```python
from build123d import *

# Parameters (mm, degrees)
SKETCH1_W           = 76.2
SKETCH1_H           = 25.4
BOSS_EXTRUDE1_DEPTH = 6.35
SKETCH2_W           = 76.2
SKETCH2_H           = 25.4
BOSS_EXTRUDE2_DEPTH = 6.35
FILLET1_R           = 3.175
FILLET2_R           = 2.3876
SKETCH3_R           = 3.3782
CUT_EXTRUDE1_DEPTH  = 7.35
SKETCH4_R           = 3.3782
CUT_EXTRUDE2_DEPTH  = 7.35


with BuildPart() as part:
    # Sketch1 → Boss-Extrude1 (new body)
    with BuildSketch(Plane(origin=(0, 0, 0), x_dir=(1, 0, 0), z_dir=(0, 1, 0))):
        with Locations((38.1, 12.7)):
            Rectangle(SKETCH1_W, SKETCH1_H)
    extrude(amount=BOSS_EXTRUDE1_DEPTH)

    # Sketch2 → Boss-Extrude2 (add)
    with BuildSketch(Plane(origin=(0, 0, -25.4), x_dir=(-1, 0, 0), z_dir=(0, 0, -1))):
        with Locations((-38.1, 12.7)):
            Rectangle(SKETCH2_W, SKETCH2_H)
    extrude(amount=-BOSS_EXTRUDE2_DEPTH)

    # Fillet1
    fillet1_edges = [part.edges().sort_by_distance(p)[0] for p in [
        (38.1, 6.35, -19.05),
    ]]
    fillet(fillet1_edges, radius=FILLET1_R)

    # Fillet2
    fillet2_edges = [part.edges().sort_by_distance(p)[0] for p in [
        (38.1, 25.4, -19.05),
        (38.1, 6.35, 0),
    ]]
    fillet(fillet2_edges, radius=FILLET2_R)

    # Sketch3 → Cut-Extrude1 (cut, through all)
    with BuildSketch(Plane(origin=(0, 6.35, 0), x_dir=(1, 0, 0), z_dir=(0, 1, 0))):
        with Locations((13.21308, 9.1313)):
            Circle(SKETCH3_R)
        with Locations((29.80436, 9.1313)):
            Circle(SKETCH3_R)
        with Locations((46.39564, 9.1313)):
            Circle(SKETCH3_R)
        with Locations((62.98692, 9.1313)):
            Circle(SKETCH3_R)
    extrude(amount=-CUT_EXTRUDE1_DEPTH, mode=Mode.SUBTRACT)

    # Sketch4 → Cut-Extrude2 (cut, through all)
    with BuildSketch(Plane.XY.offset(-19.05)):
        with Locations((13.21308, 16.2687)):
            Circle(SKETCH4_R)
        with Locations((29.80436, 16.2687)):
            Circle(SKETCH4_R)
        with Locations((46.39564, 16.2687)):
            Circle(SKETCH4_R)
        with Locations((62.98692, 16.2687)):
            Circle(SKETCH4_R)
    extrude(amount=-CUT_EXTRUDE2_DEPTH, mode=Mode.SUBTRACT)


solid = part.part
```
For this review, take the finished solid that the model builds, in its own axes (mm). A direction names the side the tool comes from. Coordinates: 2 decimals unless noted, no trailing zeros. Loops run counter-clockwise (first coordinate to the right, second up) from the corner with the lowest first, then second, coordinate; pieces in that order, holes last.
1. Add section A-A, the plane z = -11.75. Give the boundary of the cut face in (x, y), then the cut area to 3 significant figures.
2. Mouldability with a two-part tool opening along X and no side actions: class faces 3 (the flat face through (76.2, 6.9, -18.2)), 4 (the cylindrical face through (12.48, 12.97, -22.18)), 5 (the cylindrical face through (38.63, 5.67, -0.72)) as +X half, -X half, draft (parallel to the pull), parting line (faces both ways), or undercut.
3. For line 1 (Z direction, x = 42, y = 11.5); line 2 (Y direction, x = 35, z = -11.25); line 3 (Y direction, x = 11, z = -23.25), list the stretches that pass through material, from the lowest coordinate up.
4. Insertion check: P1, Ø11, axis at x = 52.5, z = -8, coming from the +Y side; P2, Ø15, axis at x = 36, y = 14.5, coming from the +Z side; P3, Ø4, axis at x = 10, y = 10.5, coming from the +Z side. Each pin has a flat end and moves straight along its axis. Give the tip position at first contact, or say it passes through.
5. Add section D-D, the plane y = 18.5. Give the boundary of the cut face in (x, z).
6. Add section C-C, the plane y = 5.25. Give the boundary of the cut face in (x, z), then the cut area to 3 significant figures.
7. Add section B-B, the plane x = 65.5. Give the boundary of the cut face in (y, z) (3 decimals), then the cut area to 3 significant figures.
8. For faces 1 (the cylindrical face through (26.43, 3.22, -9.28)), 2 (the flat face through (39, 16, -19.05)), list the 3-axis set-ups (+Z, -Z, +X, -X, +Y, -Y) from which the entire face can be reached by the end or side of a thin tool; tool diameter is ignored.
Result:
1. outline: (0, 0) - (11.08, 0) - (11.08, 6.35) - (0, 6.35) - close; (15.35, 0) - (27.67, 0) - (27.67, 6.35) - (15.35, 6.35) - close; (31.94, 0) - (44.26, 0) - (44.26, 6.35) - (31.94, 6.35) - close; (48.53, 0) - (60.85, 0) - (60.85, 6.35) - (48.53, 6.35) - close; (65.12, 0) - (76.2, 0) - (76.2, 6.35) - (65.12, 6.35) - close
1. area: 375 mm2
2. face 3: +X half
2. face 4: undercut
2. face 5: draft
3. line 1: z = -25.4 to -19.05
3. line 2: y = 0 to 6.35
3. line 3: y = 0 to 13.72, 18.82 to 25.4
4. P1: stops at y = 6.35
4. P2: stops at z = -17.8
4. P3: stops at z = -18.88
5. outline: (0, -25.4) - (10.68, -25.4) - (10.68, -19.05) - (0, -19.05) - close; (15.75, -25.4) - (27.27, -25.4) - (27.27, -19.05) - (15.75, -19.05) - close; (32.34, -25.4) - (43.86, -25.4) - (43.86, -19.05) - (32.34, -19.05) - close; (48.93, -25.4) - (60.45, -25.4) - (60.45, -19.05) - (48.93, -19.05) - close; (65.52, -25.4) - (76.2, -25.4) - (76.2, -19.05) - (65.52, -19.05) - close
6. outline: (0, -25.4) - (76.2, -25.4) - (76.2, -0.38) - (0, -0.38) - close; hole circle Ø6.76 at (13.21, -9.13); hole circle Ø6.76 at (29.8, -9.13); hole circle Ø6.76 at (46.4, -9.13); hole circle Ø6.76 at (62.99, -9.13)
6. area: 1,760 mm2
7. outline: (0, -25.4) - (14.011, -25.4) - (14.011, -19.05) - (9.525, -19.05) arc R3.175 cw to (6.35, -15.875) - (6.35, -11.389) - (0, -11.389) - close; (0, -6.874) - (6.35, -6.874) - (6.35, -2.388) arc R2.388 ccw to (3.962, 0) - (0, 0) - close; (18.526, -25.4) - (25.4, -25.4) - (25.4, -21.438) arc R2.388 ccw to (23.012, -19.05) - (18.526, -19.05) - close
7. area: 225 mm2
8. face 1: +Y, -Y
8. face 2: +Z, +X, -X, +Y
